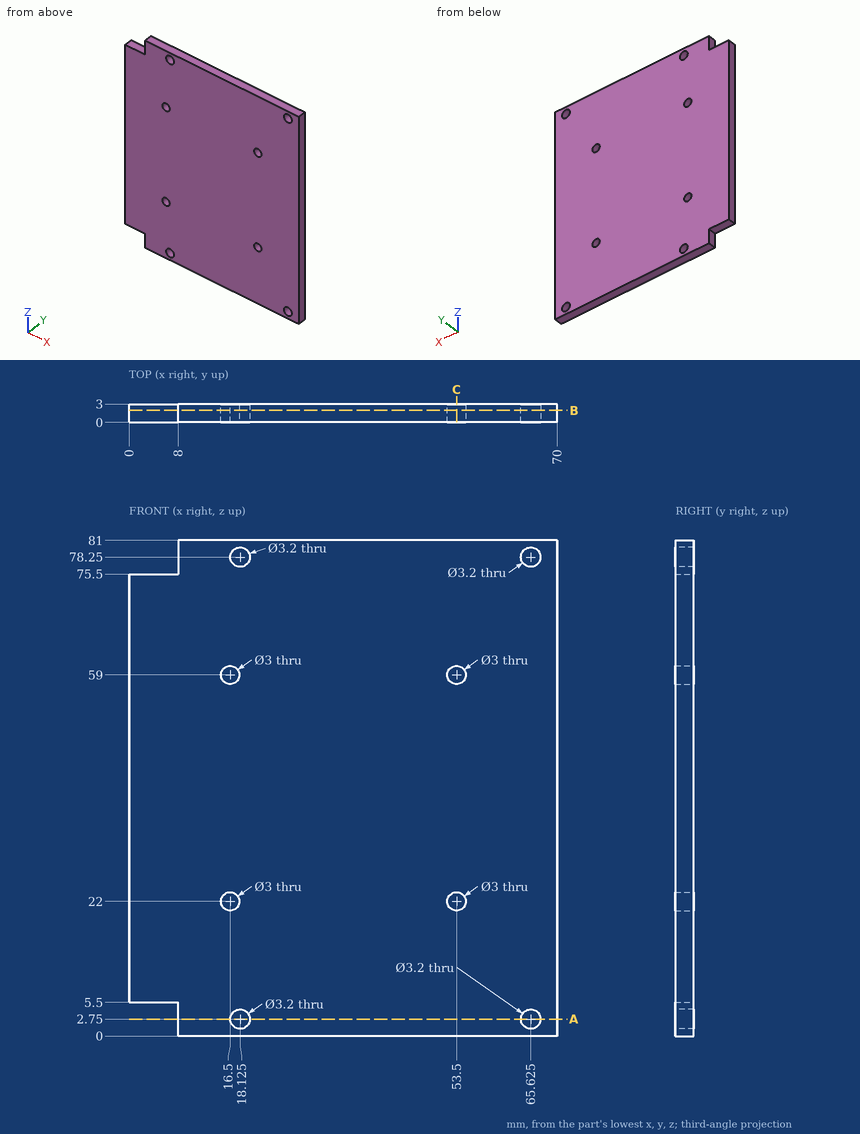
Check sheet for the drawn part. Datum: minimum x, y, z corner. Units: mm. Coordinates: 2 decimals unless noted, no trailing zeros. Order: outer loops, then holes, each group sorted by start corner. A loop starts at its lowest first (then second) coordinate and runs counter-clockwise, first axis right, second up. Notation, with made-up numbers: M -18,4.25 L -1,4.25 A25 ccw -1,24.25 Z; hole C 47,73.5 d10. An arc over 180 degrees is marked long. One line per question, with ' | ' between items. Start each with the question number.
Item 1: Sectioned sample at C-C on x = 53.5. Record the cut outline in (y, z).
Item 2: Sectioned sample at A-A on z = 2.75. Record the cut outline in (x, y) (3 decimals), and give its area (3 significant figures).
Item 3: Sectioned sample at B-B on y = 1.95. Count the separate pieces of the cut face and the enclosed holes in it, and give its area (3 significant figures).
Item 4: Material ranges on line 1 (X direction, y = 1.85, z = 78.25) (3 decimals); line 2 (X direction, y = 1.3, z = 22); line 3 (Z direction, x = 53.5, y = 0.8), recorded low to high.
Item 5: Gauge pin test, flat ends, axial feed: P1, Ø5, axis at x = 18.125, z = 78.25, coming from the -Y side; P2, Ø0.9, axis at y = 1, z = 4, coming from the -X side. Record the tip position at first contact, or that the pin passes through.
Answer below:
1) outline: M 0,0 L 3,0 L 3,20.5 L 0,20.5 Z; M 0,23.5 L 3,23.5 L 3,57.5 L 0,57.5 Z; M 0,60.5 L 3,60.5 L 3,81 L 0,81 Z
2) outline: M 8,0 L 16.525,0 L 16.525,3 L 8,3 Z; M 19.725,0 L 64.025,0 L 64.025,3 L 19.725,3 Z; M 67.225,0 L 70,0 L 70,3 L 67.225,3 Z | area: 167 mm^2
3) separate pieces: 1 | enclosed holes: 8 | area: 5,520 mm^2
4) line 1: x = 8 to 16.525, 19.725 to 64.025, 67.225 to 70 | line 2: x = 0 to 15, 18 to 52, 55 to 70 | line 3: z = 0 to 20.5, 23.5 to 57.5, 60.5 to 81
5) P1: stops at y = 0 | P2: stops at x = 8
